Here's how the part is built. I have some questions about the finished solid (model axes, mm). A direction names the side the tool comes from. Give positions to 0.01 mm unless a question says otherwise; leave off trailing zeros. Write each loop counter-clockwise with the first axis right and the second up, starting at its lowest first coordinate (ties: lowest second). Pieces come first, ordered by that corner, then holes. Notation, with made-up numbers: (-14, 67.5) - (39, 67.5) arc R26 ccw to (39, 91.5) - close; hole circle Ø10 at (8, 52). An arc over 180 degrees is marked (long way). One line per item, written item: value. Start each with the question number.
1) On a 3-axis mill with a long thin cutter (end or side, diameter ignored), from which of +Z, -Z, +X, -X, +Y, -Y can I reach the whole of each face in a straight line? I mean faces 5 (the flat face through (-18, 0, -24)), 6 (the flat face through (-15, -10, -43)). Say none if no direction works.
2) We'd pull the mould along Z, two halves only. Please class faces 1 (the cylindrical face through (-17.74, 2.54, -35.57)), 2 (the flat face through (-19, -5, -37.332)), 3 (the flat face through (-20, -3, 0)), 4 (the cylindrical face through (-26.501, -9.687, -43.249)): +Z half, -Z half, draft (parallel to the pull), parting line (faces both ways), or undercut.
3) I'm going to push flat-ended pins straight in: P1, Ø8, axis at y = -2.5, z = -12.5, coming from the -X side; P2, Ø2, axis at x = -17.11, z = -35.17, coming from the -Y side; P3, Ø0.9, axis at x = -17.11, z = -14.17, coming from the +Y side. Where does each tip first touch, or does it pass through?
4) Please list where these lines run through material, in increasing order: L1, parallel to Z at x = -29, y = -2.5; L2, parallel to Y at x = -22, z = -13.5; L3, parallel to X at y = -2.5, z = -45. Write a range as [from, to].
5) Imagine slicing it at B-B on y = -6.75. Write out the boundary of the cut face in (x, z), plus the area to 3 significant figures.
6) Imagine slicing it at A-A on x = -22.5. Write out the boundary of the cut face in (y, z), plus the area to 3 significant figures.
7) Imagine slicing it at C-C on y = 3. Write out the boundary of the cut face in (x, z).
Autodesk Inventor part; units mm, degrees
ref_plane "YZ Plane" through (0, 0, 0) normal (1, 0, 0) x (0, 1, 0)
ref_plane "XZ Plane" through (0, 0, 0) normal (0, 1, 0) x (-1, 0, 0)
ref_plane "XY Plane" through (0, 0, 0) normal (0, 0, 1) x (1, 0, 0)
sketch "Sketch1" plane through (0, 0, 0) normal (0, 1, 0) x (-1, 0, 0)
  circle A0 centre (9.758, -6.2456) radius 2.1174
  circle A1 centre (9.758, -6.2456) radius 2.1174
  circle A2 centre (9.758, -43.1772) radius 2.1174
  circle A3 centre (9.758, -43.1772) radius 2.1174
  line L0 (19.6065, 0) -> (19.6065, -49.3325)
  line L1 (19.6065, 0) -> (4.6065, 0)
  line L2 (4.6065, 0) -> (4.6065, -49.3325)
  line L3 (4.6065, -49.3325) -> (19.6065, -49.3325)
  line L4 (19.6065, -49.3325) -> (19.6065, 0)
  line L5 (4.6065, -49.3325) -> (4.6065, -54.3325)
  line L6 (19.6065, -49.3325) -> (34.6065, -49.3325)
  line L7 (34.6065, -49.3325) -> (34.6065, 0)
  line L8 (34.6065, 0) -> (19.6065, 0)
  line L9 (19.6065, 0) -> (19.6065, -49.3325)
  line L10 (34.6065, 0) -> (4.6065, -49.3325)
  line L11 (34.6065, -49.3325) -> (4.6065, 0)
  line L12 (7.6065, -37.1662) -> (31.6065, -37.1662)
  line L13 (31.6065, -37.1662) -> (31.6065, -12.1662)
  line L14 (31.6065, -12.1662) -> (7.6065, -12.1662)
  line L15 (7.6065, -12.1662) -> (7.6065, -37.1662)
  line L16 (7.6065, -37.1662) -> (31.6065, -12.1662) construction
  line L17 (31.6065, -37.1662) -> (7.6065, -12.1662) construction
  line L18 (17.1065, -14.1662) -> (29.6065, -14.1662)
  line L19 (29.6065, -14.1662) -> (29.6065, -35.1662)
  line L20 (29.6065, -35.1662) -> (17.1065, -35.1662)
  line L21 (17.1065, -35.1662) -> (17.1065, -14.1662)
  point P0 (0, 0)
  point P1 (19.6065, -49.3325)
  point P2 (-0.0904, -49.3325)
  point P3 (19.6065, -24.6662)
  dimension "d0" = 15
  dimension "d5" = 15
  dimension "d8" = 24
  dimension "d9" = 25
  dimension "d14" = 12.5
  dimension "d15" = 21
  dimension "d16" = 2
  dimension "d17" = 2
extrude "Extrusion1" add sketch "Sketch1" along normal blind 5 contours A0 L11 L1 L0 L14 | A0 L11 L14 L15 L12 L10 A2 L2 | L14 L0 L18 L21 L11 | L11 L21 L10 L12 L15 L14 | L8 L10 L14 L0 | L10 A2 L12 L0 L3 | L21 L18 L0 L11 | L11 L10 L21 | L14 L10 L18 L0 | L7 L11 L12 L13 L14 L10 | L0 L12 L11 L6 | L11 L20 L0 | L0 L18 L10 | L0 L20 L21 L10 | L10 L18 L19 L20 L11 | L21 L20 L0 L12 L10 | L14 L13 L12 L11 L20 L19 L18 L10 | L0 L20 L11 L12
hole "Hole1" at (0.0904, 0, -49.3325) at (-29.6065, 0, -35.1662) at (-29.6065, 0, -14.1662) at (-17.1065, 0, -35.1662) at (-17.1065, 0, -14.1662) direction (0, 1, 0) diameter 1.5 end through all
sketch "Sketch2" plane through (0, 0, 0) normal (0, -1, 0) x (1, 0, 0)
  line L0 (-4.6065, 0) -> (-34.6065, 0)
  line L1 (-34.6065, 0) -> (-34.6065, -12)
  line L2 (-34.6065, -12) -> (-4.6065, -12)
  line L3 (-4.6065, -12) -> (-4.6065, 0)
  line L4 (-4.6065, -49.3325) -> (-34.6065, -49.3325)
  line L5 (-34.6065, -49.3325) -> (-34.6065, -37.3325)
  line L6 (-34.6065, -37.3325) -> (-4.6065, -37.3325)
  line L7 (-4.6065, -37.3325) -> (-4.6065, -49.3325)
  point P0 (0, 0)
  dimension "d27" = 30
  dimension "d28" = 12
  dimension "d29" = 30
  dimension "d30" = 12
extrude "Extrusion2" add sketch "Sketch2" along normal blind 10
hole "Hole2" at (-9.758, 0, -6.2456) at (-9.758, 0, -43.1772) direction (0, -1, 0) diameter 4.5 end through all both
chamfer "Chamfer1" distance 8 angle 45 2 edges at (-34.6065, -10, -43.3325) (-34.6065, -10, -6)
chamfer "Chamfer2" distance 7 angle 45 2 edges at (-34.6065, -2, -43.3325) (-34.6065, -2, -6)
fillet "Fillet1" radius 4 4 edges at (-29.6574, -6.949, -6) (-26.6065, -10, -6) (-26.6065, -10, -43.3325) (-29.6574, -6.949, -43.3325)
properties part number "camera_holder"
Numbers:
1. face 5: +X, -X, -Y
1. face 6: +Z, -Z, +X, -X, -Y
2. face 1: undercut
2. face 2: undercut
2. face 3: +Z half
2. face 4: draft
3. P1: x = -33.16
3. P2: y = 0
3. P3: through
4. L1: [-49.33, -37.33], [-12, 0]
4. L2: [0, 5]
4. L3: [-31.5, -11.08], [-8.44, -4.61]
5. outline: (-29.69, -49.33) - (-4.61, -49.33) - (-4.61, -37.33) - (-29.69, -37.33) - close; (-29.69, -12) - (-4.61, -12) - (-4.61, 0) - (-29.69, 0) - close; hole circle Ø4.5 at (-9.76, -43.18); hole circle Ø4.5 at (-9.76, -6.25)
5. area: 570 mm^2
6. outline: (-10, -49.33) - (5, -49.33) - (5, 0) - (-10, 0) - (-10, -12) - (0, -12) - (0, -37.33) - (-10, -37.33) - close
6. area: 487 mm^2
7. outline: (-33.78, -49.33) - (-4.61, -49.33) - (-4.61, 0) - (-33.78, 0) - close; hole circle Ø1.5 at (-29.61, -35.17); hole circle Ø1.5 at (-29.61, -14.17); hole circle Ø1.5 at (-17.11, -35.17); hole circle Ø1.5 at (-17.11, -14.17); hole circle Ø4.5 at (-9.76, -43.18); hole circle Ø4.5 at (-9.76, -6.25)
